For this review, use the dimensioned drawing (mm, ordinates from the lowest corner) and the shaded views. A direction names the side the tool comes from. Give positions to 0.01 mm unless a question says otherwise; leave off trailing zeros. Write each loop counter-clockwise with the first axis right and the second up, starting at its lowest first coordinate (ties: lowest second). Pieces come first, ordered by that corner, then holes. Notation, with made-up numbers: (46.25, -5) -> (61.25, -5) arc R19 cw to (61.25, 5) -> close; hole circle Ø7 at (32, 58). An arc over 180 degrees is marked (long way). Return JSON: item names as keys, results as strings.
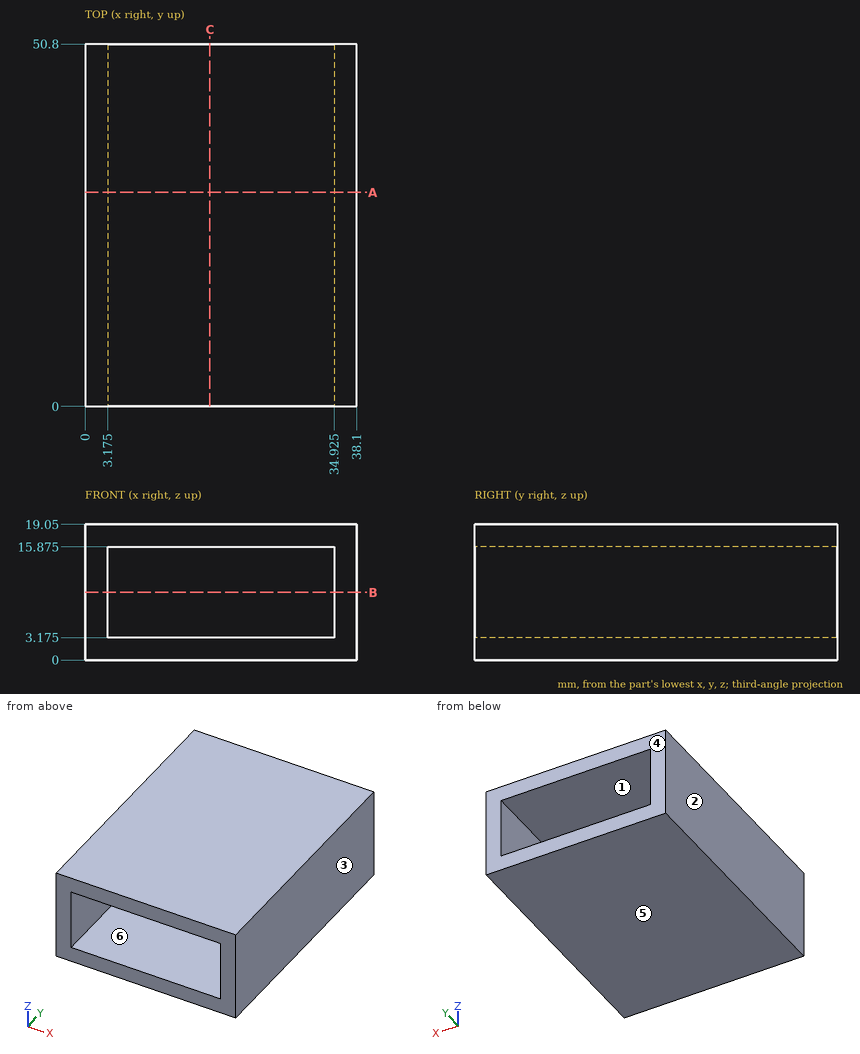
1. Add section A-A, the plane y = 30. State the section outline as (x, z) points (3 decimals), plus the area to 3 significant figures.
Results found:
{"outline": "(0, 0) -> (38.1, 0) -> (38.1, 19.05) -> (0, 19.05) -> close; hole (3.175, 3.175) -> (34.925, 3.175) -> (34.925, 15.875) -> (3.175, 15.875) -> close", "area": "323 mm²"}
2. For the marked faces 5 and 6, list the 3-axis set-ups (+Z, -Z, +X, -X, +Y, -Y) from which the entire face can be reached by the end or side of a thin tool; tool diameter is ignored.
Results found:
{"face 5": "-Z, +X, -X, +Y, -Y", "face 6": "+Y, -Y"}
3. Add section B-B, the plane z = 9.5. State the section outline as (x, y) points (3 decimals).
Results found:
{"outline": "(0, 0) -> (3.175, 0) -> (3.175, 50.8) -> (0, 50.8) -> close; (34.925, 0) -> (38.1, 0) -> (38.1, 50.8) -> (34.925, 50.8) -> close"}
4. For pin 1 (16 mm diameter, centred on x = 24, y = 30, fed in from -Z), flat-tipped, find the tip position at first contact; note if it passes through.
Results found:
{"pin 1": "stops at z = 0"}
5. To check wall thickness, follow probe 1 along X at (y, z) = (15, 7.75) (3 decimals); probe 2 along Z at (x, y) = (6.5, 45) (3 decimals). State the ranges of each line that lie inside material, in increasing order.
Results found:
{"probe 1": "x = 0 to 3.175, 34.925 to 38.1", "probe 2": "z = 0 to 3.175, 15.875 to 19.05"}
6. The part is to be moulded in two halves that separate along X. For the marked faces 1, 2, 3 and 4, say which applies: +X half, -X half, draft (parallel to the pull), parting line (faces both ways), or undercut.
Results found:
{"face 1": "undercut", "face 2": "-X half", "face 3": "+X half", "face 4": "draft"}
7. Add section C-C, the plane x = 17.5. State the section outline as (y, z) points (3 decimals), plus the area to 3 significant figures.
Results found:
{"outline": "(0, 0) -> (50.8, 0) -> (50.8, 3.175) -> (0, 3.175) -> close; (0, 15.875) -> (50.8, 15.875) -> (50.8, 19.05) -> (0, 19.05) -> close", "area": "323 mm²"}
